Verification items for the finished model (mm, model axes). Face numbers are marked on the shaded views. A direction names the side the tool comes from. Round coordinates to 2 decimals unless told otherwise and drop trailing zeros. Order: outer loops, then holes, each group sorted by start corner. A loop starts at its lowest first (then second) coordinate and runs counter-clockwise, first axis right, second up.
```python
from build123d import *

# Parameters (mm, degrees)
SKETCH1_W           = 104.14
SKETCH1_H           = 27.94
SKETCH1_R           = 2.902024653
SKETCH1_R_2         = 3.261420209
BOSS_EXTRUDE1_DEPTH = 24.13
SKETCH2_W           = 41.91
SKETCH2_H           = 20.32
CUT_EXTRUDE1_DEPTH  = 16.51
SKETCH4_W           = 24.13
SKETCH4_H           = 27.94
CUT_EXTRUDE2_DEPTH  = 16.51
FILLET1_R           = 2.54


with BuildPart() as part:
    # Sketch1 → Boss-Extrude1 (new body)
    with BuildSketch(Plane(origin=(0, 0, 0), x_dir=(1, 0, 0), z_dir=(0, 1, 0))):
        Rectangle(SKETCH1_W, SKETCH1_H)
        with Locations(Location((40.005, 0, 0), (0, 0, 90))):
            Circle(SKETCH1_R, mode=Mode.SUBTRACT)
        with Locations(Location((-40.005, 0, 0), (0, 0, 90))):
            Circle(SKETCH1_R_2, mode=Mode.SUBTRACT)
    extrude(amount=BOSS_EXTRUDE1_DEPTH)

    # Sketch2 → Cut-Extrude1 (cut)
    with BuildSketch(Plane.XZ):
        with Locations((0, 3.81)):
            Rectangle(SKETCH2_W, SKETCH2_H)
    extrude(amount=-CUT_EXTRUDE1_DEPTH, mode=Mode.SUBTRACT)

    # Sketch4 → Cut-Extrude2 (cut)
    with BuildSketch(Plane(origin=(0, 24.13, 0), x_dir=(1, 0, 0), z_dir=(0, 1, 0))):
        with Locations((-40.005, 0)):
            Rectangle(SKETCH4_W, SKETCH4_H)
        with Locations((40.005, 0)):
            Rectangle(SKETCH4_W, SKETCH4_H)
    extrude(amount=-CUT_EXTRUDE2_DEPTH, mode=Mode.SUBTRACT)

    # Fillet1
    fillet1_edges = [part.edges().sort_by_distance(p)[0] for p in [
        (-20.955, 8.255, -6.35),
        (0, 16.51, -6.35),
        (20.955, 8.255, -6.35),
        (52.07, 3.81, 13.97),
        (0, 24.13, 13.97),
        (-52.07, 3.81, 13.97),
        (-52.07, 3.81, -13.97),
        (0, 24.13, -13.97),
        (52.07, 3.81, -13.97),
        (-52.07, 7.62, 0),
        (-40.005, 7.62, -13.97),
        (-27.94, 7.62, 0),
        (-27.94, 15.875, -13.97),
        (-40.005, 7.62, 13.97),
        (-27.94, 15.875, 13.97),
        (-27.94, 24.13, 0),
        (52.07, 7.62, 0),
        (40.005, 7.62, 13.97),
        (27.94, 7.62, 0),
        (27.94, 15.875, 13.97),
        (40.005, 7.62, -13.97),
        (27.94, 15.875, -13.97),
        (27.94, 24.13, 0),
    ]]
    fillet(fillet1_edges, radius=FILLET1_R)


solid = part.part
```
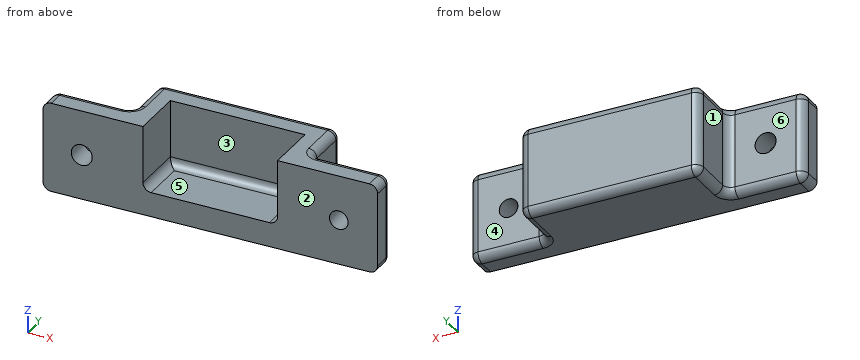
1) Draft check along X on the marked faces 1, 2 and 3. Enter one of: released by +X, released by -X, zero draft, split by the parting line, or undercut.
2) Tool access check on the marked faces 4, 5 and 6. Record the directions out of +Z, -Z, +X, -X, +Y, -Y that give a thin tool (end or side, any length) a straight path to the whole face; none if there is none.
3) Scan lines: probe 1 along X at (y, z) = (3.75, 0) (3 decimals); probe 2 along X at (y, z) = (13.5, 6.25) (3 decimals); probe 3 along Y at (x, z) = (-20, 2). Record each from-to range of solid material in increasing order.
4) Sectioned sample at A-A on z = 0. Record the cut outline in (x, y) (3 decimals).
5) Sectioned sample at C-C on z = 8.75. Record the cut outline in (x, y) (3 decimals), then the cut area to 3 significant figures.
6) Sectioned sample at B-B on x = -4. Record the cut outline in (y, z).
7) Sectioned sample at D-D on y = 18.5. Record the cut outline in (x, z), then the cut area to 3 significant figures.
8) Go/stop test with flat-tipped pins: pin 1 Ø12.5 at (y, z) = (17, -3) entering from -X; pin 2 Ø9 at (y, z) = (17, 0) entering from +X; pin 3 Ø14 at (x, z) = (-8.5, 7) entering from -Y. Record where each tip stops, or that it passes through.
Returned:
1. face 1: released by -X
1. face 2: zero draft
1. face 3: undercut
2. face 4: +Z, -Z, +X, +Y
2. face 5: +Z, -Y
2. face 6: +Z, -Z, -X, +Y
3. probe 1: x = -52.07 to -43.266, -36.744 to -20.955, 20.955 to 37.103, 42.907 to 52.07
3. probe 2: x = -27.94 to -20.955, 20.955 to 27.94
3. probe 3: y = 16.51 to 24.13
4. outline: (-52.07, 0) - (-43.266, 0) - (-43.266, 7.62) - (-49.53, 7.62) arc R2.54 ccw to (-52.07, 5.08) - close; (-36.744, 0) - (-20.955, 0) - (-20.955, 16.51) - (20.955, 16.51) - (20.955, 0) - (37.103, 0) - (37.103, 7.62) - (30.48, 7.62) arc R2.54 cw to (27.94, 10.16) - (27.94, 21.59) arc R2.54 ccw to (25.4, 24.13) - (-25.4, 24.13) arc R2.54 ccw to (-27.94, 21.59) - (-27.94, 10.16) arc R2.54 cw to (-30.48, 7.62) - (-36.744, 7.62) - close; (42.907, 0) - (52.07, 0) - (52.07, 5.08) arc R2.54 ccw to (49.53, 7.62) - (42.907, 7.62) - close
5. outline: (-52.07, 0) - (-20.955, 0) - (-20.955, 16.51) - (20.955, 16.51) - (20.955, 0) - (52.07, 0) - (52.07, 5.08) arc R2.54 ccw to (49.53, 7.62) - (30.48, 7.62) arc R2.54 cw to (27.94, 10.16) - (27.94, 21.59) arc R2.54 ccw to (25.4, 24.13) - (-25.4, 24.13) arc R2.54 ccw to (-27.94, 21.59) - (-27.94, 10.16) arc R2.54 cw to (-30.48, 7.62) - (-49.53, 7.62) arc R2.54 ccw to (-52.07, 5.08) - close
5. area: 1,020 mm2
6. outline: (0, -13.97) - (21.59, -13.97) arc R2.54 ccw to (24.13, -11.43) - (24.13, 11.43) arc R2.54 ccw to (21.59, 13.97) - (16.51, 13.97) - (16.51, -3.81) arc R2.54 cw to (13.97, -6.35) - (0, -6.35) - close
7. outline: (-27.94, -11.43) arc R2.54 ccw to (-25.4, -13.97) - (25.4, -13.97) arc R2.54 ccw to (27.94, -11.43) - (27.94, 11.43) arc R2.54 ccw to (25.4, 13.97) - (-25.4, 13.97) arc R2.54 ccw to (-27.94, 11.43) - close
7. area: 1,560 mm2
8. pin 1: stops at x = -27.94
8. pin 2: stops at x = 27.94
8. pin 3: stops at y = 16.51
